Source: CAD feature listing. Evaluate the final solid. Frame: model axes, mm. Face numbers are marked on the shaded views. Coordinates: 2 decimals unless noted, no trailing zeros.
```python
from build123d import *

# Parameters (mm, degrees)
F2_R     = 1
F3_R     = 0.5
F5_DEPTH = 1
F7_DEPTH = 3
F8_R     = 0.4


with BuildPart() as f1:
    # F0 (on Right) → F1 (revolve)
    with BuildSketch(Plane.YZ):
        Polygon((-45, 0), (0, 0), (0, 2), (-43.715038, 2), (-46, 7), (-48.198947, 7), align=None)
    revolve(axis=Axis((0, 0, 1), (0, 0, 1)))

    # F2
    f2_edges = [f1.edges().sort_by_distance(p)[0] for p in [
        (0, 45, 0),
    ]]
    fillet(f2_edges, radius=F2_R)

    # F3
    f3_edges = [f1.edges().sort_by_distance(p)[0] for p in [
        (0, 48.198947, 7),
    ]]
    fillet(f3_edges, radius=F3_R)

    # F4 (on face) → F5 (join)
    with BuildSketch(Plane.XY.offset(2)):
        with BuildLine():
            Line((1, 35), (-1, 35))
            Line((-1, 35), (-1, 3.497445))
            ThreePointArc((-1, 3.497445), (0, 2.497445), (1, 3.497445))
            Line((1, 3.497445), (1, 35))
        make_face()
        with BuildLine():
            Line((-33.595995, 9.864538), (-3.635285, 0.129714))
            ThreePointArc((-3.635285, 0.129714), (-2.375212, 0.771753), (-3.017251, 2.031827))
            Line((-3.017251, 2.031827), (-32.977961, 11.766651))
            Line((-32.977961, 11.766651), (-33.595995, 9.864538))
        make_face()
        with BuildLine():
            Line((-19.763467, -28.90338), (-1.24673, -3.417278))
            ThreePointArc((-1.24673, -3.417278), (-1.467961, -2.020476), (-2.864764, -2.241707))
            Line((-2.864764, -2.241707), (-21.381501, -27.72781))
            Line((-21.381501, -27.72781), (-19.763467, -28.90338))
        make_face()
        with BuildLine():
            Line((21.381501, -27.72781), (2.864764, -2.241707))
            ThreePointArc((2.864764, -2.241707), (1.467961, -2.020476), (1.24673, -3.417278))
            Line((1.24673, -3.417278), (19.763467, -28.90338))
            Line((19.763467, -28.90338), (21.381501, -27.72781))
        make_face()
        with BuildLine():
            Line((32.977961, 11.766651), (3.017251, 2.031827))
            ThreePointArc((3.017251, 2.031827), (2.375212, 0.771753), (3.635285, 0.129714))
            Line((3.635285, 0.129714), (33.595995, 9.864538))
            Line((33.595995, 9.864538), (32.977961, 11.766651))
        make_face()
    extrude(amount=F5_DEPTH)

    # F6 (on face) → F7 (join)
    with BuildSketch(Plane.XY.offset(2)):
        with BuildLine():
            ThreePointArc((-34.445667, 16.630049), (-22.516124, 30.920651), (-5.2535, 37.887508))
            Line((-5.2535, 37.887508), (-5.528193, 39.868554))
            ThreePointArc((-5.528193, 39.868554), (-23.693438, 32.537417), (-36.246748, 17.499594))
            Line((-36.246748, 17.499594), (-34.445667, 16.630049))
        make_face()
        with BuildLine():
            ThreePointArc((36.246553, 17.499998), (23.693076, 32.537681), (5.527749, 39.868615))
            Line((5.527749, 39.868615), (5.253078, 37.887566))
            ThreePointArc((5.253078, 37.887566), (22.51578, 30.920902), (34.445482, 16.630432))
            Line((34.445482, 16.630432), (36.246553, 17.499998))
        make_face()
        with BuildLine():
            ThreePointArc((27.781897, -29.124366), (38.239889, -12.560788), (39.640529, 6.977889))
            Line((39.640529, 6.977889), (37.670814, 6.631162))
            ThreePointArc((37.670814, 6.631162), (36.33977, -11.93665), (26.40143, -27.677193))
            Line((26.40143, -27.677193), (27.781897, -29.124366))
        make_face()
        with BuildLine():
            Line((18.8097, -35.584515), (17.875056, -33.81634))
            ThreePointArc((17.875056, -33.81634), (0, -38.25), (-17.875056, -33.81634))
            Line((-17.875056, -33.81634), (-18.8097, -35.584515))
            ThreePointArc((-18.8097, -35.584515), (0, -40.25), (18.8097, -35.584515))
        make_face()
        with BuildLine():
            ThreePointArc((-39.640607, 6.977448), (-38.239819, -12.561001), (-27.781897, -29.124366))
            Line((-27.781897, -29.124366), (-26.40143, -27.677193))
            ThreePointArc((-26.40143, -27.677193), (-36.339704, -11.936852), (-37.670887, 6.630742))
            Line((-37.670887, 6.630742), (-39.640607, 6.977448))
        make_face()
    extrude(amount=F7_DEPTH)

    # F8
    f8_edges = [f1.edges().sort_by_distance(p)[0] for p in [
        (-22.516124, 30.920651, 5),
        (-23.693438, 32.537417, 5),
        (-35.346207, 17.064821, 5),
        (-5.390846, 38.878031, 5),
        (-38.655747, 6.804095, 5),
        (-38.239819, -12.561001, 5),
        (-36.339704, -11.936852, 5),
        (-27.091664, -28.400779, 5),
        (-18.342378, -34.700427, 5),
        (0, -40.25, 5),
        (18.342378, -34.700427, 5),
        (0, -38.25, 5),
        (38.239889, -12.560788, 5),
        (36.33977, -11.93665, 5),
        (27.091664, -28.400779, 5),
        (38.655671, 6.804526, 5),
        (23.693076, 32.537681, 5),
        (35.346017, 17.065215, 5),
        (5.390413, 38.878091, 5),
        (22.51578, 30.920902, 5),
    ]]
    fillet(f8_edges, radius=F8_R)


solid = f1.part
```
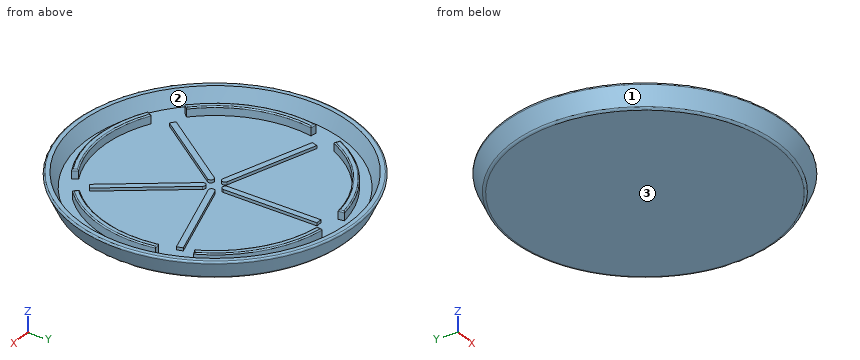
1. Material intervals for line 1 along X through (y, z) = (3.5, 4.25); line 2 along Y through (x, z) = (-29.5, 2.75); line 3 along Z through (x, y) = (-38.5, 8.5), sorted ascending.
2. Draft query along Y for the marked faces 1, 2 and 3. Return one class per face: +Y half, -Y half, draft (parallel to the pull), parting line (faces both ways), or undercut.
3. Contact query for flat-ended pins moving along their axis: P1, Ø10.5, axis at x = 34, y = -6.5, coming from the +Z side; P2, Ø0.5, axis at y = 15, z = 2.5, coming from the +X side; P3, Ø16.5, axis at x = -11.5, y = -12.5, coming from the +Z side. Output: stop coordinate, or through.
Answer key:
1. line 1: x = -46.81 to -44.61, -40.1 to -38.09, 38.09 to 40.1, 44.61 to 46.81
1. line 2: y = -35.63 to -32.72, -27.38 to -24.35, 8.53 to 10.64, 24.35 to 27.38, 32.72 to 35.63
1. line 3: z = 0 to 2
2. face 1: parting line
2. face 2: undercut
2. face 3: draft
3. P1: stops at z = 5
3. P2: stops at x = 43.78
3. P3: stops at z = 3
